CAD build for the part. Positions are in the model's coordinates, mm. Face numbers are marked on the shaded views. A direction names the side the tool comes from. Round coordinates to 2 decimals unless told otherwise and drop trailing zeros. Order: outer loops, then holes, each group sorted by start corner. A loop starts at its lowest first (then second) coordinate and runs counter-clockwise, first axis right, second up. Notation, with made-up numbers: M -1.75,-28 L 36.25,-28 A13 cw 36.25,-15 Z; hole C -27,76.5 d10. An arc over 180 degrees is marked long. Answer as a JSON object with one key per item and string values.
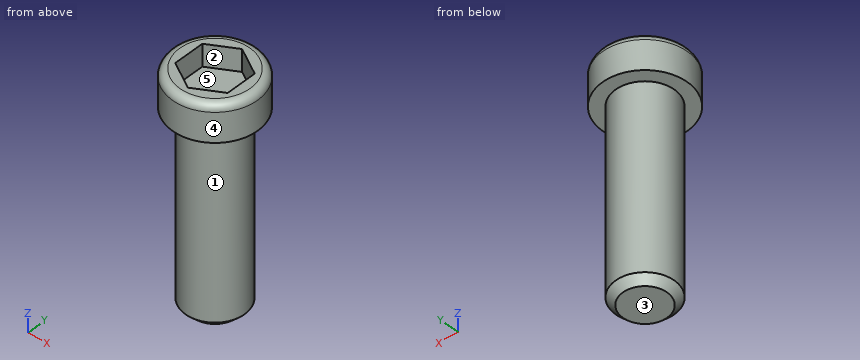
```python
from build123d import *

# Parameters (mm, degrees)
SKETCH_1_R          = 2
EXTRUDE_1_DEPTH     = 13
SKETCH_2_R          = 2.883822271
EXTRUDE_2_DEPTH     = 2.5
CUT_EXTRUDE_1_DEPTH = 1.5
CHAMFER_1_SIZE      = 0.5
FILLET_1_R          = 0.5


with BuildPart() as part:
    # 草图1 → 凸台-拉伸1 (new body)
    with BuildSketch(Plane.XY):
        with Locations(Location((0, 0, 0), (0, 0, 180))):
            Circle(SKETCH_1_R)
    extrude(amount=EXTRUDE_1_DEPTH)

    # 草图2 → 凸台-拉伸2 (add)
    with BuildSketch(Plane.XY.offset(13)):
        Circle(SKETCH_2_R)
    extrude(amount=EXTRUDE_2_DEPTH)

    # 草图3 → 切除-拉伸1 (cut)
    with BuildSketch(Plane.XY.offset(15.5)):
        Polygon((0, 2.048433274), (-1.773995253, 1.024216637), (-1.773995253, -1.024216637), (0, -2.048433274), (1.773995253, -1.024216637), (1.773995253, 1.024216637), align=None)
    extrude(amount=-CUT_EXTRUDE_1_DEPTH, mode=Mode.SUBTRACT)

    # 倒角1
    chamfer_1_edges = [part.edges().sort_by_distance(p)[0] for p in [
        (2, 0, 0),
    ]]
    chamfer(chamfer_1_edges, length=CHAMFER_1_SIZE)

    # 圆角1
    fillet_1_edges = [part.edges().sort_by_distance(p)[0] for p in [
        (-2.883822271, 0, 15.5),
    ]]
    fillet(fillet_1_edges, radius=FILLET_1_R)


solid = part.part
```
Item 1: Drop flat-ended pins along their axis: pin 1 Ø1.5 at (x, z) = (-1.5, 6.5) entering from -Y; pin 2 Ø1.5 at (y, z) = (-1.5, 10) entering from -X; pin 3 Ø1 at (x, z) = (1.5, 6) entering from -Y; pin 4 Ø1.5 at (x, y) = (-2, -0.5) entering from -Z. Give the stop position or say it passes through.
Worked answers:
{"pin 1": "stops at y = -1.85", "pin 2": "stops at x = -1.85", "pin 3": "stops at y = -1.73", "pin 4": "stops at z = 0"}
Item 2: Saw through at A-A on y = 0. List the corners of the cut face in (x, z), and give its area (3 significant figures).
Worked answers:
{"outline": "M -2.88,13 L -2,13 L -2,0.5 L -1.5,0 L 1.5,0 L 2,0.5 L 2,13 L 2.88,13 L 2.88,15 A0.5 ccw 2.38,15.5 L 1.77,15.5 L 1.77,14 L -1.77,14 L -1.77,15.5 L -2.38,15.5 A0.5 ccw -2.88,15 Z", "area": "60.7 mm2"}
Item 3: 3-axis set-ups, long thin cutter, end or side, ignore diameter. For the marked faces 1 and 2: which of +Z, -Z, +X, -X, +Y, -Y reach the whole face in a straight line?
Worked answers:
{"face 1": "-Z", "face 2": "+Z"}
Item 4: Wall check: line 1 along Z through (x, y) = (0.5, -2); line 2 along Z through (x, y) = (-1.05, 0.65); line 3 along Y through (x, z) = (0.1, 9.75). Give the ranges that are in metal, low to high. Write a range as [from, to].
Worked answers:
{"line 1": "z = [13, 15.5]", "line 2": "z = [0, 14]", "line 3": "y = [-2, 2]"}
Item 5: Saw through at B-B on z = 6.25. List the corners of the cut face in (x, y), and give its area (3 significant figures).
Worked answers:
{"outline": "C 0,0 d4", "area": "12.6 mm2"}
Item 6: Two-plate mould, pull along Y, no slides. Class the marked faces 3, 4 and 5: released by +Y, released by -Y, zero draft, split by the parting line, or undercut.
Worked answers:
{"face 3": "zero draft", "face 4": "split by the parting line", "face 5": "undercut"}
